Check sheet for the modelled part. Datum: model origin and axes. Units: mm. A direction names the side the tool comes from. Round coordinates to 2 decimals unless told otherwise and drop trailing zeros. Write each loop counter-clockwise with the first axis right and the second up, starting at its lowest first coordinate (ties: lowest second). Pieces come first, ordered by that corner, then holes. Notation, with made-up numbers: (-29.5, -10) - (18.5, -10) arc R23 ccw to (18.5, 19) - close; hole circle Ø4 at (60, 72.5). An arc over 180 degrees is marked (long way). Use one line per item in the form item = value. Start each with the question number.
1) Section check B-B (y = -164.5). Record the boundary of the cut face in (x, z).
2) Gauge pin test, flat ends, axial feed: P1, Ø6, axis at x = 58.5, y = -146, coming from the -Z side; P2, Ø10, axis at x = 54.5, y = -143, coming from the -Z side; P3, Ø8, axis at x = 57.5, y = -163, coming from the +Z side. Record the tip position at first contact, or that the pin passes through.
3) Set-up check for faces 1 (the face through (65.479, -140.77, 125.907)), 2 (the face through (81.871, -178.572, 109.082)): record each of +Z, -Z, +X, -X, +Y, -Y from which the full face is reachable in a straight line by a thin tool's end or side.
4) Scan lines: probe 1 along Z at (x, y) = (60, -147.5); probe 2 along Y at (x, z) = (85, 140.5); probe 3 along Y at (x, z) = (53.5, 157.5). Record each from-to range of solid material in increasing order.
5) Section check A-A (x = 68.5). Record the boundary of the cut face in (y, z), then the cut area to 3 significant figures.
6) Draft check along X on faces 3 (the face through (81.87, -177.12, 107.04)), 4 (the face through (82.834, -177.948, 103.215)), 5 (the face through (84.49, -180.84, 104.44)). Enter one of: +X half, -X half, draft (parallel to the pull), parting line (faces both ways), or undercut.
Autodesk Inventor part; units mm, degrees
ref_plane "YZ Plane" through (0, 0, 0) normal (1, 0, 0) x (0, 1, 0)
ref_plane "XZ Plane" through (0, 0, 0) normal (0, 1, 0) x (-1, 0, 0)
ref_plane "XY Plane" through (0, 0, 0) normal (0, 0, 1) x (1, 0, 0)
ref_plane "Work Plane1" through (87.3148, -183.736, 102.4116) normal (0, -0.5736, 0.8192) x (0, 0.8192, 0.5736)
sketch "Sketch1" plane through (87.3148, -183.736, 102.4116) normal (0, -0.5736, 0.8192) x (0, 0.8192, 0.5736)
  line L0 (96, -2.5) -> (96, 45.5)
  line L1 (0, 45.5) -> (96, 45.5)
  line L2 (0, -2.5) -> (0, 45.5)
  line L3 (-64, -2.5) -> (104, -2.5)
  circle A0 centre (-40, -26.5) radius 50.8
  circle A1 centre (88, 37.5) radius 2
  arc A2 (88.9632, 3.7472) -> (86.3648, 4.3484) centre (88, 5.5) ccw
  circle A3 centre (8, 37.5) radius 2
  circle A4 centre (8, 5.5) radius 2
  circle A5 centre (88, 5.5) radius 2
  circle A6 centre (-40, -26.5) radius 52.8
  point P0 (91.7668, 87.3148)
  point P1 (88.9632, 3.7472)
  point P2 (86.3648, 4.3484)
  dimension "d0" = 4
  dimension "d1" = 2
extrude "Extrusion1" add sketch "Sketch1" along normal blind 4 contours L3 A6 L2 L1 L0 | L3 A0 L2 A6 | L3 L2 A0 picked at (5.5904, -1.2761) picked at (0.5767, 1.5949)
sketch "Sketch2" plane through (87.3148, -186.0303, 105.6882) normal (0, -0.5736, 0.8192) x (1, 0, 0)
  line L0 (-45.5, 0) -> (2.5, 0)
  line L1 (2.5, 0) -> (2.5, 96)
  line L2 (2.5, 96) -> (-45.5, 96)
  line L3 (-45.5, 96) -> (-45.5, 0)
  circle A0 centre (-5.5, 8) radius 2
  circle A1 centre (-37.5, 8) radius 2
  circle A2 centre (-5.5, 88) radius 2
  circle A3 centre (-37.5, 88) radius 2
  circle A4 centre (26.5, -40) radius 50.8
  circle A5 centre (26.5, -40) radius 54.8
  point P0 (-87.3148, 91.7668)
  point P1 (-10.9572, 0)
  point P2 (2.5, 9.265)
  dimension "d4" = 4
extrude "Extrusion2" add sketch "Sketch2" against normal blind 9.398 contours L3 L2 L1 A5 L0 | A0
sketch "Sketch3" plane through (87.3148, -183.736, 102.4116) normal (0, 0.5736, -0.8192) x (-1, 0, 0)
  circle A0 centre (5.5, 88) radius 2
  circle A1 centre (37.5, 88) radius 2
  circle A2 centre (37.5, 8) radius 2
  circle A3 centre (5.5, 8) radius 2
  circle A4 centre (5.5, 8) radius 4
  point P0 (87.3148, 91.7668)
  dimension "d12" = 8
sketch "Sketch4" plane through (87.3148, -180.6398, 97.9899) normal (0, 0.5736, -0.8192) x (-1, 0, 0)
  circle A0 centre (5.5, 88) radius 2
  circle A1 centre (37.5, 88) radius 2
  circle A2 centre (37.5, 8) radius 2
  circle A3 centre (5.5, 88) radius 4
  circle A4 centre (37.5, 88) radius 4
  circle A5 centre (37.5, 8) radius 2
  circle A6 centre (37.5, 8) radius 4
  point P0 (87.3148, 91.7668)
  dimension "d7" = 8
  dimension "d8" = 8
  dimension "d9" = 8
extrude "Extrusion3" cut sketch "Sketch4" against normal blind 2.5 contours A0 | A1 | A2 | A3 | A4 | A6
extrude "Extrusion4" cut sketch "Sketch3" against normal blind 2.5 contours A3 | A4
properties part number "shooter spacer"
Results are:
q1.outline = (41.81, 109.29) - (89.81, 109.29) - (89.81, 120.76) - (41.81, 120.76) - close
q2.P1 = 120.14
q2.P2 = 120.84
q2.P3 = 124.62
q3.face_1 = -Z, +X, -X, +Y
q3.face_2 = none
q4.probe_1 = 121.19 to 132.67
q4.probe_2 = -136.31 to -119.93
q4.probe_3 = -112.04 to -105.11
q5.outline = (-186.03, 105.69) - (-180.64, 97.99) - (-102, 153.05) - (-107.39, 160.75) - close
q5.area = 902 mm²
q6.face_3 = undercut
q6.face_4 = +X half
q6.face_5 = draft
